from build123d import *

# Parameters (mm, degrees)
EXTRUDE_THIN1_DEPTH = 4
SKETCH4_R           = 1.5
BOSS_EXTRUDE1_DEPTH = 4
FILLET1_DEPTH       = 4
CUT_EXTRUDE2_START  = -4
CUT_EXTRUDE2_DEPTH  = 4


with BuildPart() as part:
    # Sketch1 → Extrude-Thin1 (new body)
    with BuildSketch(Plane.XY):
        Polygon((-70, 98), (-50.621778265, 98), (70, 28.358983849), (71, 30.091034656), (-50.08587988, 100), (-70, 100), align=None)
    extrude(amount=EXTRUDE_THIN1_DEPTH)

    # Sketch4 → Boss-Extrude1 (add)
    # profile 1 of 9: a face of its own
    with BuildSketch(Plane(origin=(0, 0, 0), x_dir=(-1, 0, 0), z_dir=(0, 0, -1))):
        with BuildLine():
            ThreePointArc((40.894536929, 94.982050808), (40.775277321, 95.887917465), (40.425625842, 96.732050808))
            ThreePointArc((40.425625842, 96.732050808), (35.644536929, 98.013139721), (34.363448016, 93.232050808))
            ThreePointArc((34.363448016, 93.232050808), (35.026593255, 92.40467952), (35.907068336, 91.813859338))
            Line((35.907068336, 91.813859338), (40.882005522, 94.686140662))
            ThreePointArc((40.882005522, 94.686140662), (40.891402674, 94.833963122), (40.894536929, 94.982050808))
        make_face()
        with Locations((37.394536929, 94.982050808)):
            Circle(SKETCH4_R, mode=Mode.SUBTRACT)
    # profile 2 of 9: a face of its own
    with BuildSketch(Plane(origin=(0, 0, 0), x_dir=(-1, 0, 0), z_dir=(0, 0, -1))):
        with BuildLine():
            Line((41.425625842, 95), (40.425625842, 96.732050808))
            ThreePointArc((40.425625842, 96.732050808), (40.775277321, 95.887917465), (40.894536929, 94.982050808))
            ThreePointArc((40.894536929, 94.982050808), (40.891402674, 94.833963122), (40.882005522, 94.686140662))
            Line((40.882005522, 94.686140662), (41.425625842, 95))
        make_face()
    # profile 3 of 9: a face of its own
    with BuildSketch(Plane(origin=(0, 0, 0), x_dir=(-1, 0, 0), z_dir=(0, 0, -1))):
        with BuildLine():
            ThreePointArc((35.907068336, 91.813859338), (35.026593255, 92.40467952), (34.363448016, 93.232050808))
            Line((34.363448016, 93.232050808), (35.363448016, 91.5))
            Line((35.363448016, 91.5), (35.907068336, 91.813859338))
        make_face()
    # profile 4 of 9: a face of its own
    with BuildSketch(Plane(origin=(0, 0, 0), x_dir=(-1, 0, 0), z_dir=(0, 0, -1))):
        with BuildLine():
            ThreePointArc((-9.334936491, 65.982050808), (-9.454196099, 66.887917465), (-9.803847577, 67.732050808))
            ThreePointArc((-9.803847577, 67.732050808), (-14.584936491, 69.013139721), (-15.866025404, 64.232050808))
            ThreePointArc((-15.866025404, 64.232050808), (-15.202880165, 63.40467952), (-14.322405083, 62.813859338))
            Line((-14.322405083, 62.813859338), (-9.347467898, 65.686140662))
            ThreePointArc((-9.347467898, 65.686140662), (-9.338070746, 65.833963122), (-9.334936491, 65.982050808))
        make_face()
        with Locations((-12.834936491, 65.982050808)):
            Circle(SKETCH4_R, mode=Mode.SUBTRACT)
    # profile 5 of 9: a face of its own
    with BuildSketch(Plane(origin=(0, 0, 0), x_dir=(-1, 0, 0), z_dir=(0, 0, -1))):
        with BuildLine():
            ThreePointArc((-14.322405083, 62.813859338), (-15.202880165, 63.40467952), (-15.866025404, 64.232050808))
            Line((-15.866025404, 64.232050808), (-14.866025404, 62.5))
            Line((-14.866025404, 62.5), (-14.322405083, 62.813859338))
        make_face()
    # profile 6 of 9: a face of its own
    with BuildSketch(Plane(origin=(0, 0, 0), x_dir=(-1, 0, 0), z_dir=(0, 0, -1))):
        with BuildLine():
            Line((-9.347467898, 65.686140662), (-8.803847577, 66))
            Line((-8.803847577, 66), (-9.803847577, 67.732050808))
            ThreePointArc((-9.803847577, 67.732050808), (-9.454196099, 66.887917465), (-9.334936491, 65.982050808))
            ThreePointArc((-9.334936491, 65.982050808), (-9.338070746, 65.833963122), (-9.347467898, 65.686140662))
        make_face()
    # profile 7 of 9: a face of its own
    with BuildSketch(Plane(origin=(0, 0, 0), x_dir=(-1, 0, 0), z_dir=(0, 0, -1))):
        with BuildLine():
            ThreePointArc((-59.56440991, 36.982050808), (-59.683669518, 37.887917465), (-60.033320997, 38.732050808))
            ThreePointArc((-60.033320997, 38.732050808), (-64.81440991, 40.013139721), (-66.095498823, 35.232050808))
            ThreePointArc((-66.095498823, 35.232050808), (-65.432353584, 34.40467952), (-64.551878503, 33.813859338))
            Line((-64.551878503, 33.813859338), (-59.576941317, 36.686140662))
            ThreePointArc((-59.576941317, 36.686140662), (-59.567544165, 36.833963122), (-59.56440991, 36.982050808))
        make_face()
        with Locations((-63.06440991, 36.982050808)):
            Circle(SKETCH4_R, mode=Mode.SUBTRACT)
    # profile 8 of 9: a face of its own
    with BuildSketch(Plane(origin=(0, 0, 0), x_dir=(-1, 0, 0), z_dir=(0, 0, -1))):
        with BuildLine():
            ThreePointArc((-64.551878503, 33.813859338), (-65.432353584, 34.40467952), (-66.095498823, 35.232050808))
            Line((-66.095498823, 35.232050808), (-65.095498823, 33.5))
            Line((-65.095498823, 33.5), (-64.551878503, 33.813859338))
        make_face()
    # profile 9 of 9: a face of its own
    with BuildSketch(Plane(origin=(0, 0, 0), x_dir=(-1, 0, 0), z_dir=(0, 0, -1))):
        with BuildLine():
            Line((-59.576941317, 36.686140662), (-59.033320997, 37))
            Line((-59.033320997, 37), (-60.033320997, 38.732050808))
            ThreePointArc((-60.033320997, 38.732050808), (-59.683669518, 37.887917465), (-59.56440991, 36.982050808))
            ThreePointArc((-59.56440991, 36.982050808), (-59.567544165, 36.833963122), (-59.576941317, 36.686140662))
        make_face()
    extrude(amount=-BOSS_EXTRUDE1_DEPTH)

    # Fillet1: read off the stored shape, not the designer's step
    # Fillet1 outline → Fillet1 (add)
    with BuildSketch(Plane.XY):
        with BuildLine():
            ThreePointArc((60.033320997, 38.732050808), (60.730207809, 39.590019471), (61.659897736, 40.18788074))
            ThreePointArc((61.659897736, 40.18788074), (57.09391383, 39.362702083), (52.647005809, 40.687140793))
            Line((52.647005809, 40.687140793), (59.033320997, 37))
            Line((59.033320997, 37), (60.033320997, 38.732050808))
        make_face()
        with BuildLine():
            ThreePointArc((-40.425625842, 96.732050808), (-39.72873903, 97.590019471), (-38.799049103, 98.18788074))
            ThreePointArc((-38.799049103, 98.18788074), (-43.365033009, 97.362702083), (-47.81194103, 98.687140793))
            Line((-47.81194103, 98.687140793), (-41.425625842, 95))
            Line((-41.425625842, 95), (-40.425625842, 96.732050808))
        make_face()
        with BuildLine():
            Line((-35.363448016, 91.5), (-28.977132828, 87.812859207))
            ThreePointArc((-28.977132828, 87.812859207), (-32.347584407, 91.001775167), (-33.915950681, 95.368622551))
            ThreePointArc((-33.915950681, 95.368622551), (-33.968868764, 94.264556822), (-34.363448016, 93.232050808))
            Line((-34.363448016, 93.232050808), (-35.363448016, 91.5))
        make_face()
        with BuildLine():
            ThreePointArc((9.803847577, 67.732050808), (10.500734389, 68.590019472), (11.430424316, 69.18788074))
            ThreePointArc((11.430424316, 69.18788074), (6.864440411, 68.362702083), (2.41753239, 69.687140793))
            Line((2.41753239, 69.687140793), (8.803847577, 66))
            Line((8.803847577, 66), (9.803847577, 67.732050808))
        make_face()
        with BuildLine():
            Line((14.866025404, 62.5), (21.252340591, 58.812859207))
            ThreePointArc((21.252340591, 58.812859207), (17.881889013, 62.001775167), (16.313522739, 66.368622551))
            ThreePointArc((16.313522739, 66.368622551), (16.260604656, 65.264556823), (15.866025404, 64.232050808))
            Line((15.866025404, 64.232050808), (14.866025404, 62.5))
        make_face()
        with BuildLine():
            ThreePointArc((71, 30.091034656), (67.95755311, 33.22829735), (66.543566366, 37.363456571))
            ThreePointArc((66.543566366, 37.363456571), (66.489544407, 36.262013533), (66.095498823, 35.232050808))
            Line((66.095498823, 35.232050808), (65.095498823, 33.5))
            Line((65.095498823, 33.5), (71, 30.091034656))
        make_face()
    extrude(amount=FILLET1_DEPTH)

    # Sketch5 → Cut-Extrude2 (cut)
    with BuildSketch(Plane.XY.offset(4).offset(CUT_EXTRUDE2_START)):
        with BuildLine():
            Line((71, 30.091034656), (70, 28.358983849))
            Line((70, 28.358983849), (72.530271162, 28.358983849))
            Line((72.530271162, 28.358983849), (72.530271162, 31.310199794))
            Line((72.530271162, 31.310199794), (70, 31.310199794))
            Line((70, 31.310199794), (70, 30.840200363))
            ThreePointArc((70, 30.840200363), (70.488287532, 30.449983494), (71, 30.091034656))
        make_face()
        with BuildLine():
            Line((70, 30.840200363), (70, 28.358983849))
            Line((70, 28.358983849), (71, 30.091034656))
            ThreePointArc((71, 30.091034656), (70.488287532, 30.449983494), (70, 30.840200363))
        make_face()
    extrude(amount=CUT_EXTRUDE2_DEPTH, mode=Mode.SUBTRACT)


solid = part.part
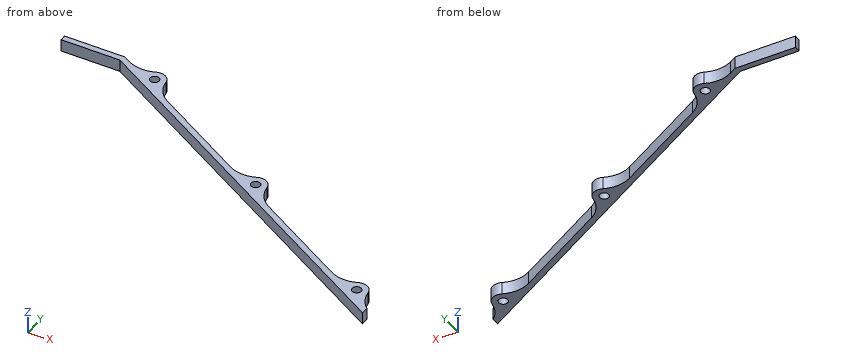
Verification items for the finished model (mm, model axes). Round coordinates to 2 decimals unless told otherwise and drop trailing zeros. Write each loop counter-clockwise with the first axis right and the second up, starting at its lowest first coordinate (ties: lowest second). Pieces come first, ordered by that corner, then holes.
(1) Material ranges on line 1 (Y direction, x = 64, z = 1.2); line 2 (Y direction, x = -52, z = 3.65); line 3 (X direction, y = 81.5, z = 0.85), recorded low to high.
Returned:
line 1: y = 31.82 to 35.81, 38.15 to 40.35
line 2: y = 98 to 100
line 3: x = -22.04 to -18.04
(2) Section check B-B (y = 90.5). Enter the section's corners in (x, z).
Returned:
outline: (-37.63, 0) - (-32, 0) - (-32, 4) - (-37.63, 4) - close
(3) Section check C-C (x = -32). Enter the section's corners in (y, z), plus the area to 3 significant figures.
Returned:
outline: (87.25, 0) - (90.5, 0) - (90.5, 4) - (87.25, 4) - close
area: 13.0 mm2
(4) Depth check by flat-ended pin: pin 1 Ø1.8 at (x, y) = (12.83, 65.98) entering from -Z; pin 2 Ø1 at (x, z) = (-14, 3) entering from +Y; pin 3 Ø2 at (x, z) = (-59, 1.5) entering from -Y; pin 4 Ø1 at (x, z) = (9.5, 3) entering from -Y. Enter the tip coordinate at first touch or a pass-through.
Returned:
pin 1: passes through
pin 2: stops at y = 79.45
pin 3: stops at y = 98
pin 4: stops at y = 63
(5) Section check A-A (z = 2.4). Enter the section's corners in (x, y), plus the area to 3 significant figures.
Returned:
outline: (-70, 98) - (-50.62, 98) - (70, 28.36) - (70, 30.84) arc R10 cw to (66.54, 37.36) arc R3.5 ccw to (61.66, 40.19) arc R10 cw to (52.65, 40.69) - (21.25, 58.81) arc R10 cw to (16.31, 66.37) arc R3.5 ccw to (11.43, 69.19) arc R10 cw to (2.42, 69.69) - (-28.98, 87.81) arc R10 cw to (-33.92, 95.37) arc R3.5 ccw to (-38.8, 98.19) arc R10 cw to (-47.81, 98.69) - (-50.09, 100) - (-70, 100) - close; hole circle Ø3 at (-37.39, 94.98); hole circle Ø3 at (12.83, 65.98); hole circle Ø3 at (63.06, 36.98)
area: 441 mm2
